Could you check a few things on this model? Use its own coordinates, in mm. A direction names the side the tool comes from. Coordinates: 2 decimals unless noted, no trailing zeros. Order: outer loops, then holes, each group sorted by start corner. A loop starts at its lowest first (then second) coordinate and runs counter-clockwise, first axis right, second up. Notation, with made-up numbers: (31, 81.25) - (63, 81.25) arc R16 ccw to (63, 91.25) - close; hole circle Ø4 at (72.25, 60). An arc over 180 degrees is marked (long way). One line per item, written item: value.
from build123d import *

# Parameters (mm, degrees)
SKETCH2_W           = 500
SKETCH2_H           = 300
SKETCH2_W_2         = 440
SKETCH2_H_2         = 240
BOSS_EXTRUDE1_DEPTH = 30
SKETCH3_W           = 30
SKETCH3_H           = 240
BOSS_EXTRUDE2_DEPTH = 30
SKETCH4_W           = 30
SKETCH4_H           = 240
BOSS_EXTRUDE3_DEPTH = 30
SKETCH8_R           = 5
CUT_EXTRUDE1_DEPTH  = 32
SKETCH9_R           = 5
CUT_EXTRUDE2_DEPTH  = 34


with BuildPart() as part:
    # Sketch2 → Boss-Extrude1 (new body)
    with BuildSketch(Plane(origin=(0, 0, 0), x_dir=(1, 0, 0), z_dir=(0, 1, 0))):
        Rectangle(SKETCH2_W, SKETCH2_H)
        Rectangle(SKETCH2_W_2, SKETCH2_H_2, mode=Mode.SUBTRACT)
    extrude(amount=BOSS_EXTRUDE1_DEPTH)

    # Sketch3 → Boss-Extrude2 (add)
    with BuildSketch(Plane(origin=(0, 30, 0), x_dir=(1, 0, 0), z_dir=(0, 1, 0))):
        Rectangle(SKETCH3_W, SKETCH3_H)
    extrude(amount=-BOSS_EXTRUDE2_DEPTH)

    # Sketch4 → Boss-Extrude3 (add)
    with BuildSketch(Plane(origin=(0, 30, 0), x_dir=(1, 0, 0), z_dir=(0, 1, 0))):
        with Locations((-99.680978572, 0)):
            Rectangle(SKETCH4_W, SKETCH4_H)
        with Locations((99.36531106, 0)):
            Rectangle(SKETCH4_W, SKETCH4_H)
    extrude(amount=-BOSS_EXTRUDE3_DEPTH)

    # Sketch8 → Cut-Extrude1 (cut)
    with BuildSketch(Plane(origin=(0, 30, 0), x_dir=(1, 0, 0), z_dir=(0, 1, 0))):
        with Locations(Location((100.018449151, 135, 0), (0, 0, 270))):
            Circle(SKETCH8_R)
    extrude(amount=-CUT_EXTRUDE1_DEPTH, mode=Mode.SUBTRACT)

    # Sketch9 → Cut-Extrude2 (cut)
    with BuildSketch(Plane(origin=(0, 30, 0), x_dir=(1, 0, 0), z_dir=(0, 1, 0))):
        with Locations(Location((100.060395289, -135, 0), (0, 0, 270))):
            Circle(SKETCH9_R)
    extrude(amount=-CUT_EXTRUDE2_DEPTH, mode=Mode.SUBTRACT)


solid = part.part
Item 1: I want a section at B-B on x = 73.5. Please give me the cut outline in (y, z), then the cut area to 3 significant figures.
Conclusion:
outline: (0, -150) - (30, -150) - (30, -120) - (0, -120) - close; (0, 120) - (30, 120) - (30, 150) - (0, 150) - close
area: 1,800 mm²
Item 2: If I drill on probe 1 along X at (y, z) = (4, -73); probe 2 along Z at (x, y) = (59, 26.5); probe 3 along X at (y, z) = (8.5, -135), over which ranges is the centre line in solid material (lowest first)?
Conclusion:
probe 1: -250 to -220, -114.68 to -84.68, -15 to 15, 84.37 to 114.37, 220 to 250
probe 2: -150 to -120, 120 to 150
probe 3: -250 to 95.02, 105.02 to 250
Item 3: For faces 4 (the face through (-3, 30, -2)), 5 (the face through (84.365, 15, 2)), which set-ups out of +Z, -Z, +X, -X, +Y, -Y let a thin tool reach every point of the face, with its end or its side?
Conclusion:
face 4: +Z, -Z, +X, -X, +Y
face 5: +Y, -Y
Item 4: Thinking about a two-plate mould opening in Z: for faces 1 (the face through (-3, 15, 150)), 2 (the face through (-3, 0, -2)), 3 (the face through (-84.681, 15, 2)), which applies, pulls with the +Z half, pulls with the -Z half, needs draft (parallel to the pull), parting line crosses it, or undercut?
Conclusion:
face 1: pulls with the +Z half
face 2: needs draft
face 3: undercut
Item 5: I want a section at C-C on z = -135. Please give me the cut outline in (x, y).
Conclusion:
outline: (-250, 0) - (95.02, 0) - (95.02, 30) - (-250, 30) - close; (105.02, 0) - (250, 0) - (250, 30) - (105.02, 30) - close
Item 6: I want a section at A-A on z = 13. Please give me the cut outline in (x, y).
Conclusion:
outline: (-250, 0) - (-220, 0) - (-220, 30) - (-250, 30) - close; (-114.68, 0) - (-84.68, 0) - (-84.68, 30) - (-114.68, 30) - close; (-15, 0) - (15, 0) - (15, 30) - (-15, 30) - close; (84.37, 0) - (114.37, 0) - (114.37, 30) - (84.37, 30) - close; (220, 0) - (250, 0) - (250, 30) - (220, 30) - close
Item 7: I want a section at D-D on y = 5. Please give me the cut outline in (x, z), then the cut area to 3 significant figures.
Conclusion:
outline: (-250, -150) - (250, -150) - (250, 150) - (-250, 150) - close; hole (-220, -120) - (-114.68, -120) - (-114.68, 120) - (-220, 120) - close; hole (-84.68, -120) - (-15, -120) - (-15, 120) - (-84.68, 120) - close; hole (15, -120) - (84.37, -120) - (84.37, 120) - (15, 120) - close; hole circle Ø10 at (100.02, -135); hole circle Ø10 at (100.06, 135); hole (114.37, -120) - (220, -120) - (220, 120) - (114.37, 120) - close
area: 65,800 mm²
